```python
from build123d import *

# Parameters (mm, degrees)
F0_W                 = 25.4
F0_H                 = 25.4
F1_DEPTH             = 25.4
F5_D                 = 6.35
F5_CBORE_D           = 10.16
F5_CBORE_DEPTH       = 19.05
F5_ON_F4_D           = 6.35
F5_ON_F4_CBORE_D     = 10.16
F5_ON_F4_CBORE_DEPTH = 19.05
F5_ON_F3_D           = 6.35
F5_ON_F3_CBORE_D     = 10.16
F5_ON_F3_CBORE_DEPTH = 19.05
F6_SIZE              = 1.905


with BuildPart() as f1:
    # F0 (on Top) → F1 (new body)
    with BuildSketch(Plane.XY):
        Rectangle(F0_W, F0_H)
    extrude(amount=F1_DEPTH)

    # F5 (through all)
    with Locations(Plane.XY.offset(25.4)):
        with Locations((0, 0)):
            CounterBoreHole(F5_D / 2, F5_CBORE_D / 2, F5_CBORE_DEPTH)

    # F5 on F4 (through all)
    with Locations(Plane(origin=(-12.7, 0, 0), x_dir=(0, -1, 0), z_dir=(-1, 0, 0))):
        with Locations((0, 12.7)):
            CounterBoreHole(F5_ON_F4_D / 2, F5_ON_F4_CBORE_D / 2, F5_ON_F4_CBORE_DEPTH)

    # F5 on F3 (through all)
    with Locations(Plane.XZ.offset(12.7)):
        with Locations((0, 12.7)):
            CounterBoreHole(F5_ON_F3_D / 2, F5_ON_F3_CBORE_D / 2, F5_ON_F3_CBORE_DEPTH)

    # F6
    f6_edges = [f1.edges().sort_by_distance(p)[0] for p in [
        (-12.7, 0, 25.4),
        (0, -12.7, 25.4),
        (-12.7, -12.7, 12.7),
    ]]
    chamfer(f6_edges, length=F6_SIZE)


solid = f1.part
```
Read the model definition and answer for the solid it produces. Units are mm, in the model's axes. A direction names the side the tool comes from. Round coordinates to 2 decimals unless told otherwise and drop trailing zeros. Write each loop counter-clockwise with the first axis right and the second up, starting at its lowest first coordinate (ties: lowest second). Pieces come first, ordered by that corner, then holes. Notation, with made-up numbers: (22, -33.5) -> (67, -33.5) arc R11 ccw to (67, -16.5) -> close; hole circle Ø10 at (32.25, -15.5). An arc over 180 degrees is marked (long way). Answer in a Markdown table with one row per item. Add a question column.
1) Which of the six approach directions +Z, -Z, +X, -X, +Y, -Y give full straight-line access (tool end or side, diameter ignored) to faces 1 (the face through (-3.744, 3.433, 7.442)), 2 (the face through (0, 6.35, 9)), 3 (the face through (-8.21, 5.075, 12.923))?
2) Find section B-B, the plane z = 12.7. Determine the outline of the cut face in (x, y) (3 decimals), and give its area (3 significant figures).
3) Determine the mould class of faces 4 (the face through (3, 3, 0)), 5 (the face through (-1.5, 9.6, 9.9)), 6 (the face through (-5.075, 0.223, 20.91)) for opening direction Z: pulls with the +Z half, pulls with the -Z half, needs draft (parallel to the pull), parting line crosses it, or undercut.
4) Find section D-D, the plane z = 5.75. Determine the outline of the cut face in (x, y) (3 decimals).
5) Consider line 1 (Y direction, x = -5.5, z = 12.7); line 2 (Z direction, x = -1.25, y = -3). Determine where each line is inside the solid, lowest interval first.
6) Given P1, Ø10, axis at y = 0, z = 12.7, coming from the -X side; P2, Ø11, axis at x = -0.5, y = -2, coming from the +Z side; P3, Ø8.5, axis at x = 0, y = 0, coming from the +Z side; P4, Ø8, axis at x = 0, z = 12.7, coming from the -Y side, each flat-ended and moving along its own axis, determine where each tip first touches the part or whether it passes through.
7) Find section C-C, the plane y = 8. Determine the outline of the cut face in (x, z) (3 decimals), and give its area (3 significant figures).
8) Find section A-A, the plane y = 0. Determine the outline of the cut face in (x, z) (3 decimals).
Findings below:
| question | item | result |
|---|---|---|
| 1 | face 1 | +Z |
| 1 | face 2 | -Y |
| 1 | face 3 | -X |
| 2 | outline | (-12.7, -10.795) -> (-10.795, -12.7) -> (-5.08, -12.7) -> (-5.08, -5.08) -> (-12.7, -5.08) -> close; (-12.7, 5.08) -> (-5.08, 5.08) -> (-5.08, 6.35) -> (-3.175, 6.35) -> (-3.175, 12.7) -> (-12.7, 12.7) -> close; (3.175, 6.35) -> (5.08, 6.35) -> (5.08, 5.08) -> (6.35, 5.08) -> (6.35, 3.175) -> (12.7, 3.175) -> (12.7, 12.7) -> (3.175, 12.7) -> close; (5.08, -12.7) -> (12.7, -12.7) -> (12.7, -3.175) -> (6.35, -3.175) -> (6.35, -5.08) -> (5.08, -5.08) -> close |
| 2 | area | 279 mm² |
| 3 | face 4 | pulls with the -Z half |
| 3 | face 5 | undercut |
| 3 | face 6 | needs draft |
| 4 | outline | (-12.7, -10.795) -> (-10.795, -12.7) -> (12.7, -12.7) -> (12.7, 12.7) -> (-12.7, 12.7) -> close; hole circle Ø6.35 at (0, 0) |
| 5 | line 1 | -12.7 to -5.08, 5.08 to 12.7 |
| 5 | line 2 | 0 to 6.35 |
| 6 | P1 | x = 6.35 |
| 6 | P2 | z = 25.4 |
| 6 | P3 | z = 6.35 |
| 6 | P4 | y = 6.35 |
| 7 | outline | (-12.7, 0) -> (12.7, 0) -> (12.7, 25.4) -> (-10.795, 25.4) -> (-12.7, 23.495) -> close; hole circle Ø6.35 at (0, 12.7) |
| 7 | area | 612 mm² |
| 8 | outline | (-12.7, 0) -> (-3.175, 0) -> (-3.175, 6.35) -> (-5.08, 6.35) -> (-5.08, 7.62) -> (-12.7, 7.62) -> close; (-12.7, 17.78) -> (-5.08, 17.78) -> (-5.08, 25.4) -> (-10.795, 25.4) -> (-12.7, 23.495) -> close; (3.175, 0) -> (12.7, 0) -> (12.7, 9.525) -> (6.35, 9.525) -> (6.35, 7.62) -> (5.08, 7.62) -> (5.08, 6.35) -> (3.175, 6.35) -> close; (5.08, 17.78) -> (6.35, 17.78) -> (6.35, 15.875) -> (12.7, 15.875) -> (12.7, 25.4) -> (5.08, 25.4) -> close |
